Input: part model. Units: mm. Frame: model coordinates. A direction names the side the tool comes from. Give positions to 0.01 mm unless a question says otherwise; leave off trailing zeros. Order: outer loops, then holes, each group sorted by start corner. A loop starts at its lowest first (then second) coordinate and runs counter-clockwise, first axis right, second up. Notation, with made-up numbers: (-32, -9) - (23, -9) arc R21 ccw to (23, 12) - close; hole circle Ø9 at (-0.5, 29.5). An arc over 180 degrees is marked (long way). Answer in a Markdown table with one row per item. Add a question column.
1. Section query A-A on x = -12. Return loops of the section in (y, z), and give its area (3 significant figures).
2. Ray query, line 1 (X direction, y = -32.05, z = 3.75); line 2 (Y direction, x = 12, z = 6.5); line 3 (Y direction, x = -12.5, z = 4.25). Return the intervals inside material, ascending. Write a range as [from, to].
3. Section query D-D on x = -18. Return loops of the section in (y, z).
4. Mould query, pull axis Y, two halves, no side actions, for faces 3 (the face through (-13.11, 19.01, 3.7)), 4 (the face through (0, 23, 4)), 5 (the face through (6, -30, 4)), 6 (the face through (10.89, -16.99, 3.7)). Classes: released by +Y, released by -Y, zero draft, split by the parting line, or undercut.
5. Contact query for a flat-ended pin moving along its axis: pin 1 (0.9 mm diameter, centred on x = -6, z = 3.5, fed in from -Y). Output: stop coordinate, or through.
6. Section query B-B on y = -18. Return loops of the section in (x, z), and give its area (3 significant figures).
7. Section query C-C on z = 3.75. Return loops of the section in (x, y), and give its area (3 significant figures).
8. Access query for faces 1 (the face through (-13.11, -16.99, 3.7)), 2 (the face through (-6, -30, 4)). Directions: +Z, -Z, +X, -X, +Y, -Y. A direction counts if a zero-diameter tool reaches every point of the face in a straight line with its end or side. Return the directions, or none.
```python
from build123d import *

# Parameters (mm, degrees)
SKETCH_1_W          = 44
SKETCH_1_H          = 56
SKETCH_1_R          = 1.5
EXTRUDE_1_DEPTH     = 7.5
SKETCH_2_R          = 1.5
CUT_EXTRUDE_1_DEPTH = 3


with BuildPart() as part:
    # 草圖1 → 填料-伸長1 (new body)
    with BuildSketch(Plane.XY):
        with Locations((0, -5)):
            Rectangle(SKETCH_1_W, SKETCH_1_H)
        with Locations((-12, 18)):
            Circle(SKETCH_1_R, mode=Mode.SUBTRACT)
        with Locations((12, 18)):
            Circle(SKETCH_1_R, mode=Mode.SUBTRACT)
        with Locations((12, -18)):
            Circle(SKETCH_1_R, mode=Mode.SUBTRACT)
        with Locations((-12, -18)):
            Circle(SKETCH_1_R, mode=Mode.SUBTRACT)
    extrude(amount=EXTRUDE_1_DEPTH)

    # 草圖2 → 除料-伸長1 (cut)
    with BuildSketch(Plane(origin=(0, -33, 0), x_dir=(-1, 0, 0), z_dir=(0, -1, 0))):
        with Locations(Location((-6, -3.75, 0), (0, 0, 90))):
            Circle(SKETCH_2_R)
        with Locations(Location((-18, -3.75, 0), (0, 0, 90))):
            Circle(SKETCH_2_R)
        with Locations(Location((6, -3.75, 0), (0, 0, 90))):
            Circle(SKETCH_2_R)
        with Locations(Location((18, -3.75, 0), (0, 0, 90))):
            Circle(SKETCH_2_R)
    extrude(amount=-CUT_EXTRUDE_1_DEPTH, mode=Mode.SUBTRACT)


solid = part.part
```
Answer:
| question | item | result |
|---|---|---|
| 1 | outline | (-33, 0) - (-19.5, 0) - (-19.5, 7.5) - (-33, 7.5) - close; (-16.5, 0) - (16.5, 0) - (16.5, 7.5) - (-16.5, 7.5) - close; (19.5, 0) - (23, 0) - (23, 7.5) - (19.5, 7.5) - close |
| 1 | area | 375 mm² |
| 2 | line 1 | x = [-22, -19.5], [-16.5, -7.5], [-4.5, 4.5], [7.5, 16.5], [19.5, 22] |
| 2 | line 2 | y = [-33, -19.5], [-16.5, 16.5], [19.5, 23] |
| 2 | line 3 | y = [-33, -19.41], [-16.59, 16.59], [19.41, 23] |
| 3 | outline | (-33, 0) - (23, 0) - (23, 7.5) - (-33, 7.5) - (-33, 5.25) - (-30, 5.25) - (-30, 2.25) - (-33, 2.25) - close |
| 4 | face 3 | undercut |
| 4 | face 4 | released by +Y |
| 4 | face 5 | released by -Y |
| 4 | face 6 | undercut |
| 5 | pin 1 | stops at y = -30 |
| 6 | outline | (-22, 0) - (-13.5, 0) - (-13.5, 7.5) - (-22, 7.5) - close; (-10.5, 0) - (10.5, 0) - (10.5, 7.5) - (-10.5, 7.5) - close; (13.5, 0) - (22, 0) - (22, 7.5) - (13.5, 7.5) - close |
| 6 | area | 285 mm² |
| 7 | outline | (-22, -33) - (-19.5, -33) - (-19.5, -30) - (-16.5, -30) - (-16.5, -33) - (-7.5, -33) - (-7.5, -30) - (-4.5, -30) - (-4.5, -33) - (4.5, -33) - (4.5, -30) - (7.5, -30) - (7.5, -33) - (16.5, -33) - (16.5, -30) - (19.5, -30) - (19.5, -33) - (22, -33) - (22, 23) - (-22, 23) - close; hole circle Ø3 at (-12, -18); hole circle Ø3 at (-12, 18); hole circle Ø3 at (12, -18); hole circle Ø3 at (12, 18) |
| 7 | area | 2,400 mm² |
| 8 | face 1 | +Z, -Z |
| 8 | face 2 | -Y |
